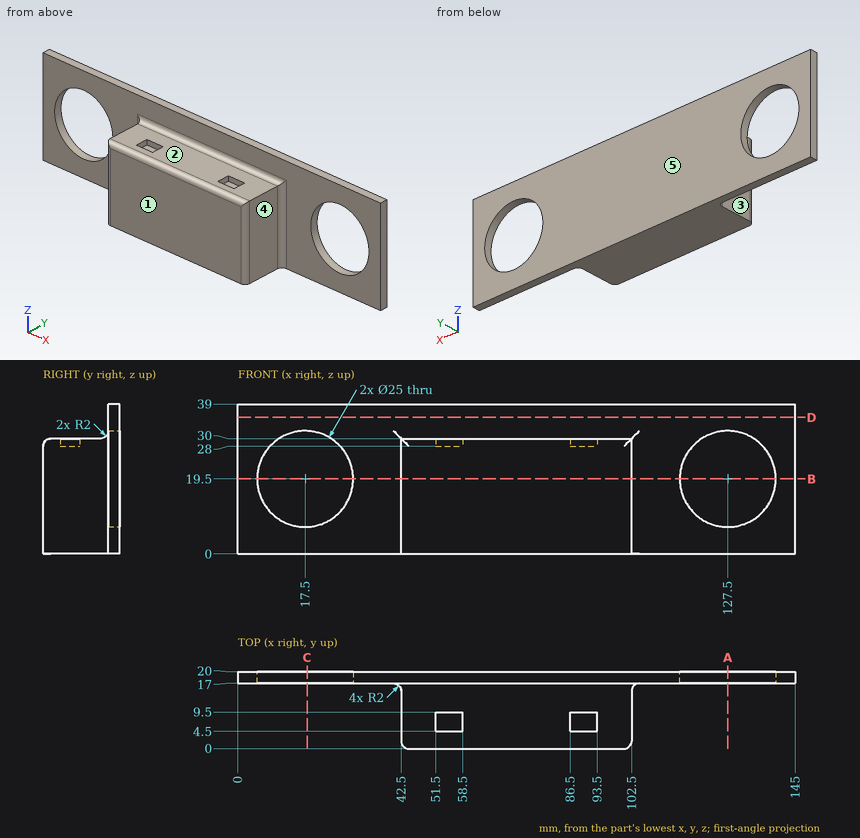
Job drawing, mm, ordinate dimensions from the low corner. One solid piece. A direction names the side the tool comes from. Give positions to 0.01 mm unless a question says otherwise; leave off trailing zeros. Loops run counter-clockwise (first coordinate to the right, second up) from the corner with the lowest first, then second, coordinate; pieces in that order, holes last. Notation, with made-up numbers: M -40,63.25 L -13,63.25 A24 ccw -13,89.25 Z; hole C -28.5,35.25 d9. An arc over 180 degrees is marked long. Return JSON: item names as keys, results as strings.
1) Saw through at C-C, the plane x = 18. List the corners of the cut face in (y, z), then the cut area to 3 significant figures.
Calculated:
{"outline": "M 17,0 L 20,0 L 20,7.01 L 17,7.01 Z; M 17,31.99 L 20,31.99 L 20,39 L 17,39 Z", "area": "42.1 mm2"}
2) Drill centre lines: line 1 (Z direction, x = 127.5, y = 18.2); line 2 (X direction, y = 17.5, z = 22.5); line 3 (X direction, y = 18.75, z = 18). Where is each one in solid material? Low to high.
Calculated:
{"line 1": "z = 0 to 7, 32 to 39", "line 2": "x = 0 to 5.37, 29.63 to 115.37, 139.63 to 145", "line 3": "x = 0 to 5.09, 29.91 to 115.09, 139.91 to 145"}
3) Flat gauge pins, fed straight in: pin 1 Ø2 at (y, z) = (7, 29) entering from -X; pin 2 Ø15 at (x, z) = (17.5, 19.5) entering from -Y; pin 3 Ø6 at (y, z) = (9.5, 32.5) entering from +X; pin 4 Ø2.5 at (x, y) = (89.5, 8) entering from +Z. Where does each tip first touch, or does it go through?
Calculated:
{"pin 1": "stops at x = 42.5", "pin 2": "passes through", "pin 3": "stops at x = 102.5", "pin 4": "stops at z = 28"}
4) 3-axis set-ups, long thin cutter, end or side, ignore diameter. For the marked faces 1, 2, 3, 4 and 5: which of +Z, -Z, +X, -X, +Y, -Y reach the whole face in a straight line?
Calculated:
{"face 1": "+Z, -Z, +X, -X, -Y", "face 2": "+Z, +X, -X, -Y", "face 3": "+Z, -Z, -X, -Y", "face 4": "+Z, -Z, +X, -Y", "face 5": "+Z, -Z, +X, -X, +Y"}
5) Saw through at D-D, the plane z = 35.5. List the corners of the cut face in (x, y), then the cut area to 3 significant figures.
Calculated:
{"outline": "M 0,17 L 145,17 L 145,20 L 0,20 Z", "area": "435 mm2"}
6) Saw through at B-B, the plane z = 19.5. List the corners of the cut face in (x, y), then the cut area to 4 significant figures.
Calculated:
{"outline": "M 0,17 L 5,17 L 5,20 L 0,20 Z; M 30,17 L 40.5,17 A2 cw 42.5,15 L 42.5,2 A2 ccw 44.5,0 L 100.5,0 A2 ccw 102.5,2 L 102.5,15 A2 cw 104.5,17 L 115,17 L 115,20 L 30,20 Z; M 140,17 L 145,17 L 145,20 L 140,20 Z", "area": "1,305 mm2"}
7) Saw through at A-A, the plane x = 127.5. List the corners of the cut face in (y, z).
Calculated:
{"outline": "M 17,0 L 20,0 L 20,7 L 17,7 Z; M 17,32 L 20,32 L 20,39 L 17,39 Z"}
